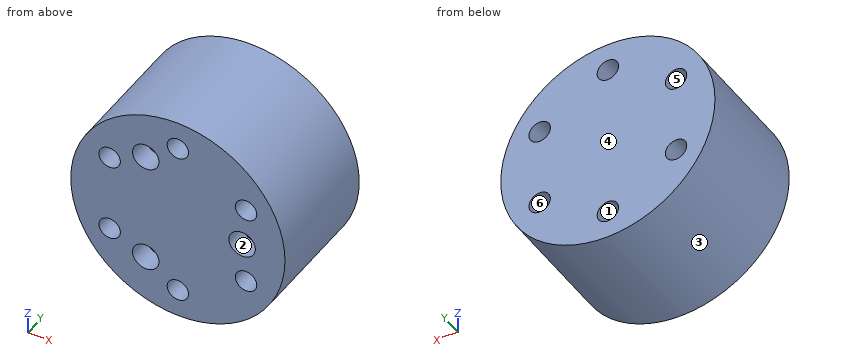
```python
from build123d import *

# Parameters (mm, degrees)
CUBO_START            = 40.25
SK_CUBO_R             = 17
CUBO_DEPTH            = 19.5
PASANTES_M3_START     = 40.25
SK_PASANTES_M3_R      = 1.7
PASANTES_M3_DEPTH     = 19.5
PASADORES_MOTOR_START = 40.25
SK_PASADORES_MOTOR_R  = 2.1
PASADORES_MOTOR_DEPTH = 3.5


with BuildPart() as part:
    # Sk_Cubo → Cubo (new body)
    with BuildSketch(Plane(origin=(0, 0, 0), x_dir=(1, 0, 0), z_dir=(0, 1, 0)).offset(CUBO_START)):
        with Locations(Location((0, -330, 0), (0, 0, 270))):
            Circle(SK_CUBO_R)
    extrude(amount=CUBO_DEPTH)

    # Sk_Pasantes_M3 → Pasantes_M3 (cut)
    with BuildSketch(Plane(origin=(0, 0, 0), x_dir=(1, 0, 0), z_dir=(0, 1, 0)).offset(PASANTES_M3_START)):
        with Locations(Location((10.825317547, -336.25, 0), (0, 0, 270))):
            Circle(SK_PASANTES_M3_R)
        with Locations(Location((0, -342.5, 0), (0, 0, 270))):
            Circle(SK_PASANTES_M3_R)
        with Locations(Location((-10.825317547, -336.25, 0), (0, 0, 270))):
            Circle(SK_PASANTES_M3_R)
        with Locations(Location((-10.825317547, -323.75, 0), (0, 0, 270))):
            Circle(SK_PASANTES_M3_R)
        with Locations(Location((0, -317.5, 0), (0, 0, 270))):
            Circle(SK_PASANTES_M3_R)
        with Locations(Location((10.825317547, -323.75, 0), (0, 0, 270))):
            Circle(SK_PASANTES_M3_R)
    extrude(amount=PASANTES_M3_DEPTH, mode=Mode.SUBTRACT)

    # Sk_Pasadores_motor → Pasadores_motor (cut)
    with BuildSketch(Plane(origin=(0, 0, 0), x_dir=(1, 0, 0), z_dir=(0, 1, 0)).offset(PASADORES_MOTOR_START)):
        with Locations(Location((10.2, -330, 0), (0, 0, 270))):
            Circle(SK_PASADORES_MOTOR_R)
        with Locations(Location((-5.1, -338.833459119, 0), (0, 0, 270))):
            Circle(SK_PASADORES_MOTOR_R)
        with Locations(Location((-5.1, -321.166540881, 0), (0, 0, 270))):
            Circle(SK_PASADORES_MOTOR_R)
    extrude(amount=PASADORES_MOTOR_DEPTH, mode=Mode.SUBTRACT)


solid = part.part
```
Input: part model. Units: mm. Frame: model coordinates. Face numbers are marked on the shaded views. A direction names the side the tool comes from. Round coordinates to 2 decimals unless told otherwise and drop trailing zeros. Loops run counter-clockwise (first coordinate to the right, second up) from the corner with the lowest first, then second, coordinate; pieces in that order, holes last. Notation, with made-up numbers: M 79,60 L 95,60 A17 ccw 95,92 Z; hole C -3,58.25 d9. An arc over 180 degrees is marked long. Answer in a Markdown table with one row per item. Add a question column.
1. Section D-D (y = 52.5). Output: boundary loops of the cut face in (x, z), and give its area (3 significant figures).
2. Section C-C (z = 336.25). Output: boundary loops of the cut face in (x, y).
3. Contact query for flat-ended pins moving along their axis: pin 1 (6 mm diameter, centred on y = 51.5, z = 333.5, fed in from -X); pin 2 (1.3 mm diameter, centred on x = 10.5, z = 329.5, fed in from -Y); pin 3 (6 mm diameter, centred on y = 57.5, z = 322, fed in from +X). Output: stop coordinate, or through.
4. Ray query, probe 1 along Z at (x, y) = (-1.5, 47); probe 2 along Z at (x, y) = (12, 45.75); probe 3 along X at (y, z) = (47, 336). Return the intervals inside material, ascending.
5. Section B-B (z = 318). Output: boundary loops of the cut face in (x, y), and give its area (3 significant figures).
6. Mould query, pull axis Z, two halves, no side actions, for the marked faces 3, 4, 5 and 6. Classes: released by +Z, released by -Z, zero draft, split by the parting line, or undercut.
7. Set-up query: the marked faces 1 and 2. Return all of +Z, -Z, +X, -X, +Y, -Y with unobstructed straight access to the full face (end or side cutting, diameter ignored); none if empty.
8. Section A-A (x = 10.2). Output: boundary loops of the cut face in (y, z), and give its area (3 significant figures).
Values follow:
| question | item | result |
|---|---|---|
| 1 | outline | C 0,330 d34; hole C -10.83,323.75 d3.4; hole C -10.83,336.25 d3.4; hole C 0,317.5 d3.4; hole C 0,342.5 d3.4; hole C 10.83,323.75 d3.4; hole C 10.83,336.25 d3.4 |
| 1 | area | 853 mm^2 |
| 2 | outline | M -15.81,40.25 L -12.53,40.25 L -12.53,59.75 L -15.81,59.75 Z; M -9.13,40.25 L 9.13,40.25 L 9.13,59.75 L -9.13,59.75 Z; M 12.53,40.25 L 15.81,40.25 L 15.81,59.75 L 12.53,59.75 Z |
| 3 | pin 1 | x = -16.99 |
| 3 | pin 2 | y = 43.75 |
| 3 | pin 3 | x = 16.25 |
| 4 | probe 1 | 313.07 to 316.7, 318.3 to 341.7, 343.3 to 346.93 |
| 4 | probe 2 | 317.96 to 322.52, 324.98 to 335.02, 337.48 to 342.04 |
| 4 | probe 3 | -15.91 to -12.51, -9.14 to 9.14, 12.51 to 15.91 |
| 5 | outline | M -12.04,40.25 L -1.62,40.25 L -1.62,59.75 L -12.04,59.75 Z; M 1.62,40.25 L 12.04,40.25 L 12.04,59.75 L 1.62,59.75 Z |
| 5 | area | 406 mm^2 |
| 6 | face 3 | split by the parting line |
| 6 | face 4 | zero draft |
| 6 | face 5 | undercut |
| 6 | face 6 | undercut |
| 7 | face 1 | +Y, -Y |
| 7 | face 2 | -Y |
| 8 | outline | M 40.25,316.4 L 59.75,316.4 L 59.75,322.17 L 40.25,322.17 Z; M 40.25,325.33 L 59.75,325.33 L 59.75,334.67 L 40.25,334.67 L 40.25,332.1 L 43.75,332.1 L 43.75,327.9 L 40.25,327.9 Z; M 40.25,337.83 L 59.75,337.83 L 59.75,343.6 L 40.25,343.6 Z |
| 8 | area | 392 mm^2 |
